```python
from build123d import *

# Parameters (mm, degrees)
SKETCH1_R           = 12.5
BOSS_EXTRUDE1_DEPTH = 37.5
SKETCH4_R           = 17.5
BOSS_EXTRUDE3_DEPTH = 5


with BuildPart() as part:
    # Sketch1 → Boss-Extrude1 (new body, symmetric)
    with BuildSketch(Plane(origin=(0, 0, 0), x_dir=(0, 0, -1), z_dir=(1, 0, 0))):
        Circle(SKETCH1_R)
    extrude(amount=BOSS_EXTRUDE1_DEPTH, both=True)

    # Sketch4 → Boss-Extrude3 (add)
    with BuildSketch(Plane(origin=(37.5, 0, 0), x_dir=(0, 0, -1), z_dir=(1, 0, 0))):
        Circle(SKETCH4_R)
    boss_extrude3 = extrude(amount=BOSS_EXTRUDE3_DEPTH)

    # Mirror1: Boss-Extrude3 across plane
    add(boss_extrude3.mirror(Plane(origin=(0, 0, 0), x_dir=(0, 0, 1), z_dir=(1, 0, 0))))


solid = part.part
```
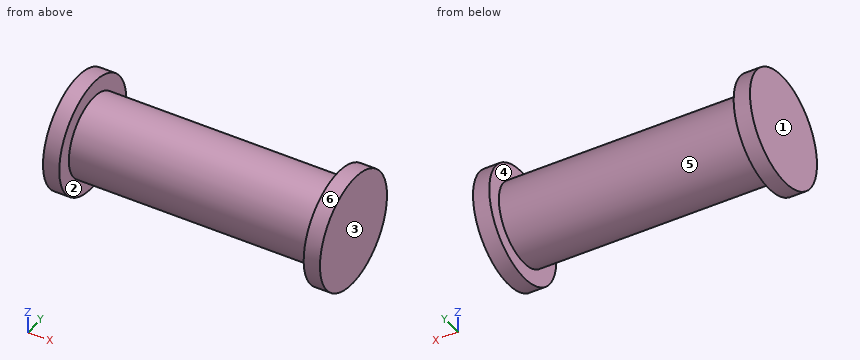
The listing builds one solid part. Answer for the finished solid, in the listing's coordinates (mm). Face numbers are marked on the shaded views. A direction names the side the tool comes from. Round coordinates to 2 decimals unless told otherwise and drop trailing zeros. Loops run counter-clockwise (first coordinate to the right, second up) from the corner with the lowest first, then second, coordinate; pieces in that order, holes last.
Q1. Given pin 1 Ø8 at (x, y) = (33, 3) entering from -Z; pin 2 Ø3 at (x, z) = (-24.5, 5.5) entering from +Y; pin 3 Ø3 at (x, z) = (4, 7.5) entering from -Y, each flat-ended and moving along its own axis, determine where each tip first touches the part or whether it passes through.
Q2. Section B-B, the plane z = 0 is taken. Determine the outline of the cut face in (x, y), then the cut area to 4 significant figures.
Q3. Section A-A, the plane y = 15 is taken. Determine the outline of the cut face in (x, z).
Q4. Which of the six approach directions +Z, -Z, +X, -X, +Y, -Y give full straight-line access (tool end or side, diameter ignored) to the marked faces 5 and 6?
Q5. Find the intervals of material crossed by line 1 (X direction, y = 9.5, z = -12.5); line 2 (Z direction, x = -34.5, y = 8.5); line 3 (Y direction, x = -25, z = 7), in increasing order.
Q6. For a pull along X with two mould halves and no side action, classify the marked faces 1, 2, 3 and 4 as released by +X, released by -X, zero draft, split by the parting line, or undercut.
Completed:
1. pin 1: stops at z = -12.5
1. pin 2: stops at y = 11.84
1. pin 3: stops at y = -10.97
2. outline: (-42.5, -17.5) - (-37.5, -17.5) - (-37.5, -12.5) - (37.5, -12.5) - (37.5, -17.5) - (42.5, -17.5) - (42.5, 17.5) - (37.5, 17.5) - (37.5, 12.5) - (-37.5, 12.5) - (-37.5, 17.5) - (-42.5, 17.5) - close
2. area: 2,225 mm2
3. outline: (-42.5, -9.01) - (-37.5, -9.01) - (-37.5, 9.01) - (-42.5, 9.01) - close; (37.5, -9.01) - (42.5, -9.01) - (42.5, 9.01) - (37.5, 9.01) - close
4. face 5: none
4. face 6: +X, -X
5. line 1: x = -42.5 to -37.5, 37.5 to 42.5
5. line 2: z = -9.17 to 9.17
5. line 3: y = -10.36 to 10.36
6. face 1: released by -X
6. face 2: undercut
6. face 3: released by +X
6. face 4: undercut
